Geometry check sheet. Reference: drawing and pictorial views, mm from the part's lowest x, y, z. A direction names the side the tool comes from. Round coordinates to 2 decimals unless told otherwise and drop trailing zeros. Write each loop counter-clockwise with the first axis right and the second up, starting at its lowest first coordinate (ties: lowest second). Pieces come first, ordered by that corner, then holes. Notation, with made-up numbers: M 86.5,17.5 L 90.5,17.5 A13 cw 90.5,22.5 Z; hole C 37.5,31.25 d9. An arc over 180 degrees is marked long. Answer in a Markdown table with one row per item. Add a question column.
1. Draft check along Y on the marked faces 3, 4 and 5. Enter one of: pulls with the +Y half, pulls with the -Y half, needs draft (parallel to the pull), parting line crosses it, or undercut.
2. Sectioned sample at A-A on x = 3.9. Record the cut outline in (y, z).
3. Go/stop test with flat-tipped pins: pin 1 Ø3 at (y, z) = (2.5, 6) entering from +X; pin 2 Ø1.4 at (x, z) = (5, 4.5) entering from -Y; pin 3 Ø1.6 at (x, y) = (3.9, 2.5) entering from -Z; pin 4 Ø2.5 at (x, y) = (3.9, 2.5) entering from +Z. Record where each tip stops, or that it passes through.
4. Material ranges on probe 1 along Z at (x, y) = (3.9, 1.3); probe 2 along X at (y, z) = (4.25, 2); probe 3 along Y at (x, z) = (5.75, 5), recorded low to high.
5. Sectioned sample at B-B on y = 2.5. Record the cut outline in (x, z), plus the area to 3 significant figures.
6. Sectioned sample at C-C on z = 3.9. Record the cut outline in (x, y), plus the area to 3 significant figures.
7. Sectioned sample at D-D on y = 4.25. Record the cut outline in (x, z).
8. Set-up check for the marked faces 1 and 2: record each of +Z, -Z, +X, -X, +Y, -Y from which the full face is reachable in a straight line by a thin tool's end or side.
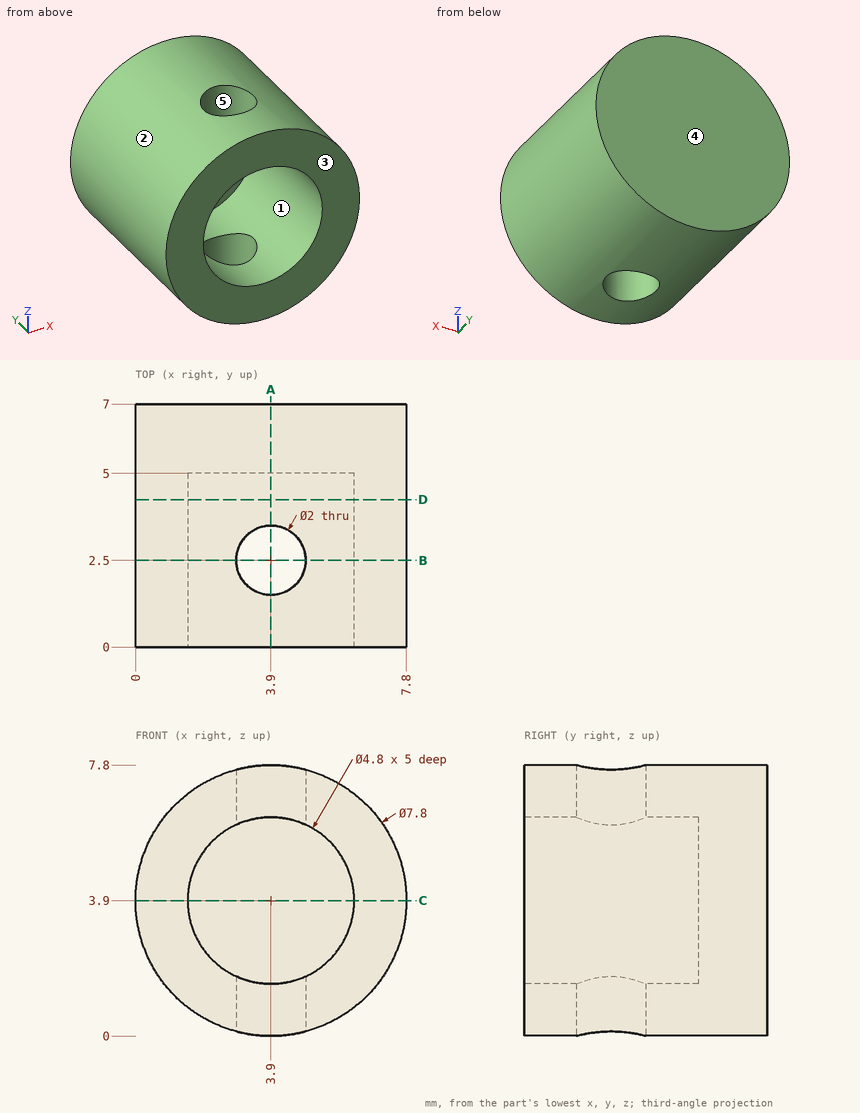
Geometry check:
| question | item | result |
|---|---|---|
| 1 | face 3 | pulls with the -Y half |
| 1 | face 4 | pulls with the +Y half |
| 1 | face 5 | undercut |
| 2 | outline | M 0,0 L 1.5,0 L 1.5,1.5 L 0,1.5 Z; M 0,6.3 L 1.5,6.3 L 1.5,7.8 L 0,7.8 Z; M 3.5,0 L 7,0 L 7,7.8 L 3.5,7.8 L 3.5,6.3 L 5,6.3 L 5,1.5 L 3.5,1.5 Z |
| 3 | pin 1 | stops at x = 7.75 |
| 3 | pin 2 | stops at y = 5 |
| 3 | pin 3 | passes through |
| 3 | pin 4 | stops at z = 7.8 |
| 4 | probe 1 | z = 0 to 1.5, 6.3 to 7.8 |
| 4 | probe 2 | x = 0.49 to 2.43, 5.37 to 7.31 |
| 4 | probe 3 | y = 5 to 7 |
| 5 | outline | M 2.9,0.13 L 2.9,1.72 A2.4 cw 2.9,6.08 L 2.9,7.67 A3.9 ccw Z; M 4.9,0.13 A3.9 ccw 4.9,7.67 L 4.9,6.08 A2.4 cw 4.9,1.72 Z |
| 5 | area | 23.6 mm2 |
| 6 | outline | M 0,0 L 1.5,0 L 1.5,5 L 6.3,5 L 6.3,0 L 7.8,0 L 7.8,7 L 0,7 Z |
| 6 | area | 30.6 mm2 |
| 7 | outline | C 3.9,3.9 d7.8; hole C 3.9,3.9 d4.8 |
| 8 | face 1 | -Y |
| 8 | face 2 | +Y, -Y |
